from build123d import *

# Parameters (mm, degrees)
ESBO_O3_W                = 30
ESBO_O3_H                = 29
ESBO_O3_R                = 1.5
RESSALTO_EXTRUS_O2_DEPTH = 4
ESBO_O5_W                = 30
ESBO_O5_H                = 14.6
CORTE_EXTRUS_O2_DEPTH    = 2


with BuildPart() as part:
    # Esboço3 → Ressalto-extrusão2 (new body)
    with BuildSketch(Plane.XY):
        with Locations((0, 8)):
            Rectangle(ESBO_O3_W, ESBO_O3_H)
        with Locations((-12.5, 19.897915762)):
            Circle(ESBO_O3_R, mode=Mode.SUBTRACT)
        with Locations((-7, 17.5)):
            Circle(ESBO_O3_R, mode=Mode.SUBTRACT)
        with Locations((12, 4.5)):
            Circle(ESBO_O3_R, mode=Mode.SUBTRACT)
        with Locations((7, 17.5)):
            Circle(ESBO_O3_R, mode=Mode.SUBTRACT)
        with Locations((12.5, 19.897915762)):
            Circle(ESBO_O3_R, mode=Mode.SUBTRACT)
    extrude(amount=RESSALTO_EXTRUS_O2_DEPTH)

    # Esboço5 → Corte-extrusão2 (cut)
    with BuildSketch(Plane(origin=(0, 0, 0), x_dir=(-1, 0, 0), z_dir=(0, 0, -1))):
        with Locations((0, 0.8)):
            Rectangle(ESBO_O5_W, ESBO_O5_H)
    extrude(amount=-CORTE_EXTRUS_O2_DEPTH, mode=Mode.SUBTRACT)


solid = part.part
The listing builds one solid part. Answer for the finished solid, in the listing's coordinates (mm). A direction names the side the tool comes from. Round coordinates to 2 decimals unless told otherwise and drop trailing zeros. Write each loop counter-clockwise with the first axis right and the second up, starting at its lowest first coordinate (ties: lowest second). Pieces come first, ordered by that corner, then holes. Notation, with made-up numbers: (-9, 32) - (20, 32) arc R32 ccw to (20, 63) - close; hole circle Ø10 at (50, 21). An arc over 180 degrees is marked (long way). Use one line per item in the form item = value. Start each with the question number.
Item 1: A cutting plane is placed at B-B (x = -12.5). Write down the section's boundary in (y, z).
Item 2: Flat-ended cylindrical pins translate along their axes: pin 1 Ø7.5 at (x, y) = (6.5, -1.5) entering from -Z; pin 2 Ø0.6 at (x, z) = (2.5, 1.5) entering from -Y. Find the tip coordinate at first contact, or state that the pin passes through.
Item 3: A cutting plane is placed at D-D (z = 2.4). Write down the section's boundary in (x, y), plus the area to 3 significant figures.
Item 4: A tool of negligible diameter and unlimited length cuts with its end or side. For faces 1 (the flat face through (0, 1, 2)), 2 (the cylindrical face through (-8.11, 18.51, 1.97)), from which of +Z, -Z, +X, -X, +Y, -Y can it reach the whole face along a straight path? Write none if from no direction.
Item 5: Find the intervals of material crossed by line 1 (Y direction, x = -12.5, z = 3); line 2 (Y direction, x = 7, z = 2.75); line 3 (Z direction, x = 0.5, y = -3.25), in increasing order. Write a range as [from, to].
Item 6: A cutting plane is placed at C-C (y = 17.5). Write down the section's boundary in (x, z).
Item 7: Determine the mould class of faces 3 (the cylindrical face through (5.89, 18.51, 1.97)), 4 (the cylindrical face through (13.31, 21.16, 1.97)), 5 (the flat face through (-15, 11, 2)), 6 (the flat face through (0, -6.5, 3)) for opening direction X: +X half, -X half, draft (parallel to the pull), parting line (faces both ways), or undercut.
Item 8: A cutting plane is placed at A-A (y = 4.5). Write down the section's boundary in (x, z).
The answers:
q1.outline = (-6.5, 2) - (8.1, 2) - (8.1, 0) - (18.4, 0) - (18.4, 4) - (-6.5, 4) - close; (21.4, 0) - (22.5, 0) - (22.5, 4) - (21.4, 4) - close
q2.pin_1 = 2
q2.pin_2 = 8.1
q3.outline = (-15, -6.5) - (15, -6.5) - (15, 22.5) - (-15, 22.5) - close; hole circle Ø3 at (-12.5, 19.9); hole circle Ø3 at (-7, 17.5); hole circle Ø3 at (7, 17.5); hole circle Ø3 at (12, 4.5); hole circle Ø3 at (12.5, 19.9)
q3.area = 835 mm^2
q4.face_1 = -Z, +X, -X, -Y
q4.face_2 = +Z, -Z
q5.line_1 = [-6.5, 18.4], [21.4, 22.5]
q5.line_2 = [-6.5, 16], [19, 22.5]
q5.line_3 = [2, 4]
q6.outline = (-15, 0) - (-8.5, 0) - (-8.5, 4) - (-15, 4) - close; (-5.5, 0) - (5.5, 0) - (5.5, 4) - (-5.5, 4) - close; (8.5, 0) - (15, 0) - (15, 4) - (8.5, 4) - close
q7.face_3 = undercut
q7.face_4 = undercut
q7.face_5 = -X half
q7.face_6 = draft
q8.outline = (-15, 2) - (10.5, 2) - (10.5, 4) - (-15, 4) - close; (13.5, 2) - (15, 2) - (15, 4) - (13.5, 4) - close
